```python
from build123d import *

# Parameters (mm, degrees)
F0_W     = 19.05
F0_H     = 88.9
F1_DEPTH = 609.6
F3_DEPTH = 88.901
F5_DEPTH = 19.05


with BuildPart() as f1:
    # F0 (on Front) → F1 (new body)
    with BuildSketch(Plane.XZ):
        Rectangle(F0_W, F0_H)
    extrude(amount=F1_DEPTH)

    # F2 (on face) → F3 (cut, through all)
    with BuildSketch(Plane.XY.offset(44.45)):
        Polygon((9.525, -590.55), (-9.525, -609.6), (9.525, -609.6), align=None)
        Polygon((9.525, 0), (-9.525, 0), (9.525, -19.05), align=None)
    extrude(amount=-F3_DEPTH, mode=Mode.SUBTRACT)

    # F4 (on face) → F5 (cut)
    with BuildSketch(Plane.XY.offset(44.45)):
        Polygon((0, -9.525), (0, -600.075), (9.525, -590.55), (9.525, -19.05), align=None)
    extrude(amount=-F5_DEPTH, mode=Mode.SUBTRACT)


solid = f1.part
```
Geometry check sheet. Reference: the model listing, model coordinates, mm. A direction names the side the tool comes from. Give positions to 0.01 mm unless a question says otherwise; leave off trailing zeros. Write each loop counter-clockwise with the first axis right and the second up, starting at its lowest first coordinate (ties: lowest second). Pieces come first, ordered by that corner, then holes. Notation, with made-up numbers: (32.25, -0.75) -> (43.25, -0.75) arc R23 ccw to (43.25, 29.25) -> close; hole circle Ø4 at (3, -30). An arc over 180 degrees is marked (long way). One line per question, with ' | ' between items.
Item 1: Access from +Z, -Z, +X, -X, +Y, -Y to the whole of each face (thin tool, end or side, straight path). Record for faces 1 (the flat face through (0, -301, 35)), 2 (the flat face through (-9.525, -301, -1)).
Determined:
face 1: +Z, +X, +Y, -Y | face 2: +Z, -Z, -X, +Y, -Y
Item 2: Scan lines: line 1 along Z through (x, y) = (6.25, -538); line 2 along X through (y, z) = (-50, 36) (3 decimals); line 3 along Y through (x, z) = (7.5, -31) (3 decimals). Record each from-to range of solid material in increasing order.
Determined:
line 1: -44.45 to 25.4 | line 2: -9.525 to 0 | line 3: -592.575 to -17.025
Item 3: Depth check by flat-ended pin: pin 1 (4 mm diameter, centred on x = 7.5, z = -10, fed in from -Y) (3 decimals); pin 2 (10 mm diameter, centred on x = -4.5, z = 32.5, fed in from +Y) (3 decimals); pin 3 (1.5 mm diameter, centred on x = -7.5, z = -30, fed in from +Y) (3 decimals). Enter the tip coordinate at first touch or a pass-through.
Determined:
pin 1: y = -594.575 | pin 2: y = -0.025 | pin 3: y = -1.275
Item 4: Sectioned sample at C-C, the plane x = 4. Record the boundary of the cut face in (y, z) (3 decimals).
Determined:
outline: (-596.075, -44.45) -> (-13.525, -44.45) -> (-13.525, 25.4) -> (-596.075, 25.4) -> close
Item 5: Sectioned sample at B-B, the plane z = 3. Record the boundary of the cut face in (x, y) (3 decimals), plus the area to 4 significant figures.
Determined:
outline: (-9.525, -609.6) -> (9.525, -590.55) -> (9.525, -19.05) -> (-9.525, 0) -> close | area: 11,250 mm^2
Item 6: Sectioned sample at A-A, the plane y = -539. Record the boundary of the cut face in (x, z) (3 decimals), plus the area to 3 significant figures.
Determined:
outline: (-9.525, -44.45) -> (9.525, -44.45) -> (9.525, 25.4) -> (0, 25.4) -> (0, 44.45) -> (-9.525, 44.45) -> close | area: 1,510 mm^2
